Can you work these out from the model? Positions are in its coordinate system, mm. Face numbers are marked on the shaded views. A direction names the side the tool comes from. Give positions to 0.01 mm unless a question says otherwise; leave off trailing zeros. Write each loop counter-clockwise with the first axis right and the second up, starting at its lowest first coordinate (ties: lowest second). Pieces come first, ordered by that corner, then holes. Notation, with made-up numbers: (28.25, 64) -> (86.25, 64) arc R32 ccw to (86.25, 102) -> close; hole circle Ø11 at (-7, 49.25). An arc over 180 degrees is marked (long way). One line per item, written item: value.
from build123d import *

# Parameters (mm, degrees)
F1_DEPTH = 1.2
F3_DEPTH = 23.8


with BuildPart() as f1:
    # F0 (on Top) → F1 (new body)
    with BuildSketch(Plane.XY):
        with BuildLine():
            ThreePointArc((170, 90.5), (155.355339, 125.855339), (120, 140.5))
            Line((120, 140.5), (-120, 140.5))
            ThreePointArc((-120, 140.5), (-155.355339, 125.855339), (-170, 90.5))
            Line((-170, 90.5), (-170, -90.5))
            ThreePointArc((-170, -90.5), (-155.355339, -125.855339), (-120, -140.5))
            Line((-120, -140.5), (120, -140.5))
            ThreePointArc((120, -140.5), (155.355339, -125.855339), (170, -90.5))
            Line((170, -90.5), (170, 90.5))
        make_face()
        with BuildLine():
            ThreePointArc((120, 120.5), (141.213203, 111.713203), (150, 90.5))
            Line((150, 90.5), (150, -90.5))
            ThreePointArc((150, -90.5), (141.213203, -111.713203), (120, -120.5))
            Line((120, -120.5), (-120, -120.5))
            ThreePointArc((-120, -120.5), (-141.213203, -111.713203), (-150, -90.5))
            Line((-150, -90.5), (-150, 90.5))
            ThreePointArc((-150, 90.5), (-141.213203, 111.713203), (-120, 120.5))
            Line((-120, 120.5), (120, 120.5))
        make_face(mode=Mode.SUBTRACT)
    extrude(amount=F1_DEPTH)

    # F2 (on face) → F3 (join)
    with BuildSketch(Plane(origin=(0, 0, 0), x_dir=(1, 0, 0), z_dir=(0, 0, -1))):
        with BuildLine():
            ThreePointArc((120, -121.7), (142.061732, -112.561732), (151.2, -90.5))
            Line((151.2, -90.5), (151.2, 90.5))
            ThreePointArc((151.2, 90.5), (142.061732, 112.561732), (120, 121.7))
            Line((120, 121.7), (-120, 121.7))
            ThreePointArc((-120, 121.7), (-142.061732, 112.561732), (-151.2, 90.5))
            Line((-151.2, 90.5), (-151.2, -90.5))
            ThreePointArc((-151.2, -90.5), (-142.061732, -112.561732), (-120, -121.7))
            Line((-120, -121.7), (120, -121.7))
        make_face()
        with BuildLine():
            ThreePointArc((150, -90.5), (141.213203, -111.713203), (120, -120.5))
            Line((120, -120.5), (-120, -120.5))
            ThreePointArc((-120, -120.5), (-141.213203, -111.713203), (-150, -90.5))
            Line((-150, -90.5), (-150, 90.5))
            ThreePointArc((-150, 90.5), (-141.213203, 111.713203), (-120, 120.5))
            Line((-120, 120.5), (120, 120.5))
            ThreePointArc((120, 120.5), (141.213203, 111.713203), (150, 90.5))
            Line((150, 90.5), (150, -90.5))
        make_face(mode=Mode.SUBTRACT)
    extrude(amount=F3_DEPTH)


solid = f1.part
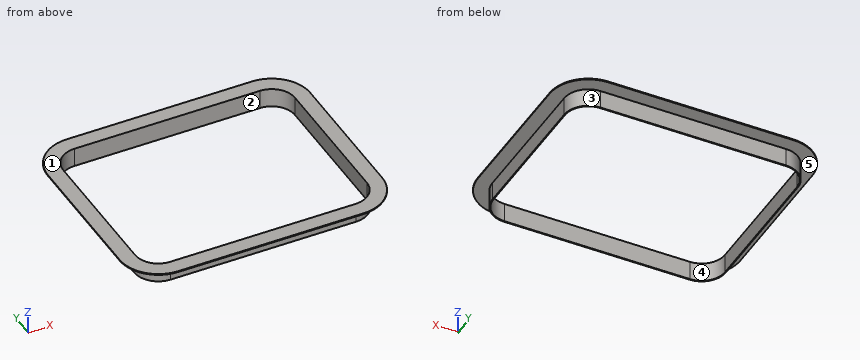
1) If we section it at C-C (z = -6.5): Write out the boundary of the cut face in (x, y), and give its area (3 significant figures).
Answer list:
outline: (-151.2, -90.5) arc R31.2 ccw to (-120, -121.7) -> (120, -121.7) arc R31.2 ccw to (151.2, -90.5) -> (151.2, 90.5) arc R31.2 ccw to (120, 121.7) -> (-120, 121.7) arc R31.2 ccw to (-151.2, 90.5) -> close; hole (-150, -90.5) arc R30 ccw to (-120, -120.5) -> (120, -120.5) arc R30 ccw to (150, -90.5) -> (150, 90.5) arc R30 ccw to (120, 120.5) -> (-120, 120.5) arc R30 ccw to (-150, 90.5) -> close
area: 1,240 mm^2
2) If we section it at B-B (x = 63.5): Write out the boundary of the cut face in (y, z), and give its area (3 significant figures).
Answer list:
outline: (-140.5, 0) -> (-121.7, 0) -> (-121.7, -23.8) -> (-120.5, -23.8) -> (-120.5, 1.2) -> (-140.5, 1.2) -> close; (120.5, -23.8) -> (121.7, -23.8) -> (121.7, 0) -> (140.5, 0) -> (140.5, 1.2) -> (120.5, 1.2) -> close
area: 105 mm^2
3) I need wall thicknesses on L1, parallel to Y at x = 118, z = -18.75; L2, parallel to X at y = -82, z = -20.25; L3, parallel to X at y = 117, z = -0.75. Which ranges of each line are inside material? Lowest first, please.
Answer list:
L1: y = -121.7 to -120.5, 120.5 to 121.7
L2: x = -151.2 to -150, 150 to 151.2
L3: x = -136.47 to -134.06, 134.06 to 136.47
4) We'd pull the mould along X, two halves only. Please class the marked faces 1, 2 and 3: released by +X, released by -X, zero draft, split by the parting line, or undercut.
Answer list:
face 1: zero draft
face 2: undercut
face 3: released by +X
5) If we section it at A-A (y = -86): Write out the boundary of the cut face in (x, z).
Answer list:
outline: (-170, 0) -> (-151.2, 0) -> (-151.2, -23.8) -> (-150, -23.8) -> (-150, 1.2) -> (-170, 1.2) -> close; (150, -23.8) -> (151.2, -23.8) -> (151.2, 0) -> (170, 0) -> (170, 1.2) -> (150, 1.2) -> close
6) For the marked faces 4 and 5, which set-ups out of +Z, -Z, +X, -X, +Y, -Y let a thin tool reach every point of the face, with its end or its side?
Answer list:
face 4: +Z, -Z
face 5: -Z
7) Will these pins go through, and if not, where does the flat tip stop? pin 1 (1 mm diameter, centred on y = -69.5, z = -8, fed in from +X); pin 2 (3 mm diameter, centred on x = 32, z = -13, fed in from +Y); pin 3 (7 mm diameter, centred on y = -14, z = -13.5, fed in from -X).
Answer list:
pin 1: stops at x = 151.2
pin 2: stops at y = 121.7
pin 3: stops at x = -151.2
